```python
from build123d import *

# Parameters (mm, degrees)
CYLINDER052_R             = 1.5
CYLINDER052_DEPTH         = 10
CYLINDER048_R             = 31
CYLINDER048_DEPTH         = 6
CYLINDER047_R             = 36
CYLINDER047_DEPTH         = 3
FUSION025_PLACEMENT_ANGLE = 180


with BuildPart() as cylinder052:
    # Cylinder052 → Cylinder052 (new body)
    with BuildSketch(Plane(origin=(39, 45.2, 83), x_dir=(1, 0, 0), z_dir=(0, 0, 1))):
        Circle(CYLINDER052_R)
    extrude(amount=CYLINDER052_DEPTH)


with BuildPart() as cylinder048:
    # Cylinder048 → Cylinder048 (new body)
    with BuildSketch(Plane.XY):
        Circle(CYLINDER048_R)
    extrude(amount=CYLINDER048_DEPTH)


with BuildPart() as cap:
    # Cylinder047 → Cylinder047 (new body)
    with BuildSketch(Plane.XY):
        Circle(CYLINDER047_R)
    extrude(amount=CYLINDER047_DEPTH)

    # Fusion025: union Cylinder048
    add(cylinder048.part)


with BuildPart() as cap_1:
    # Fusion025 placement: moved
    add(cap.part.moved(Location((39, 45.2, 90))).rotate(Axis((39, 45.2, 90), (1, 0, 0)), FUSION025_PLACEMENT_ANGLE))

    # Cut055: cut Cylinder052
    add(cylinder052.part, mode=Mode.SUBTRACT)


solid = cap_1.part
```
Model file for the job. Use its own axes, mm. A direction names the side the tool comes from. Coordinates: 2 decimals unless noted, no trailing zeros. Order: outer loops, then holes, each group sorted by start corner. A loop starts at its lowest first (then second) coordinate and runs counter-clockwise, first axis right, second up. Notation, with made-up numbers: (-11, 86.25) -> (20, 86.25) arc R29 cw to (20, 121.25) -> close; hole circle Ø6 at (-28, 52.5). An arc over 180 degrees is marked (long way). Answer as a JSON object with one key per item and string values. Group by question number.
1) Which spindle directions (+Z, -Z, +X, -X, +Y, -Y) get a long thin tool onto all of the face, cutting with end or side? Do faces 1 (the face through (46, 45, 90)), 2 (the face through (32.28, 75.463, 85.521)). Say none if no direction does.
2) Flat gauge pins, fed straight in: pin 1 (1.8 mm diameter, centred on x = 39, y = 45.2, fed in from -Z); pin 2 (1 mm diameter, centred on x = 53.5, z = 87.5, fed in from -Y). Where does each tip first touch, or does it go through?
3) Cut at C-C, the plane z = 85.1. Write the cut outline in (x, y), then the cut area to 3 significant figures.
4) Cut at B-B, the plane x = 39. Write the cut outline in (y, z), then the cut area to 3 significant figures.
5) Cut at A-A, the plane y = 45.2. Write the cut outline in (x, z).
6) Drill centre lines: L1, parallel to Y at x = 39, z = 88.75; L2, parallel to X at y = 45.2, z = 87.95; L3, parallel to Y at x = 39, z = 85.8. Where is each one in solid material? Low to high.
7) Cut at D-D, the plane x = 50.5. Write the cut outline in (y, z), then the cut area to 3 significant figures.
Check values:
{
 "1": {"face 1": "+Z, +X, -X, +Y, -Y", "face 2": "-Z"},
 "2": {"pin 1": "passes through", "pin 2": "stops at y = 12.03"},
 "3": {"outline": "circle Ø62 at (39, 45.2); hole circle Ø3 at (39, 45.2)", "area": "3,010 mm²"},
 "4": {"outline": "(9.2, 87) -> (14.2, 87) -> (14.2, 84) -> (43.7, 84) -> (43.7, 90) -> (9.2, 90) -> close; (46.7, 84) -> (76.2, 84) -> (76.2, 87) -> (81.2, 87) -> (81.2, 90) -> (46.7, 90) -> close", "area": "384 mm²"},
 "5": {"outline": "(3, 87) -> (8, 87) -> (8, 84) -> (37.5, 84) -> (37.5, 90) -> (3, 90) -> close; (40.5, 84) -> (70, 84) -> (70, 87) -> (75, 87) -> (75, 90) -> (40.5, 90) -> close"},
 "6": {"L1": "y = 9.2 to 43.7, 46.7 to 81.2", "L2": "x = 3 to 37.5, 40.5 to 75", "L3": "y = 14.2 to 43.7, 46.7 to 76.2"},
 "7": {"outline": "(11.09, 87) -> (16.41, 87) -> (16.41, 84) -> (73.99, 84) -> (73.99, 87) -> (79.31, 87) -> (79.31, 90) -> (11.09, 90) -> close", "area": "377 mm²"}
}
